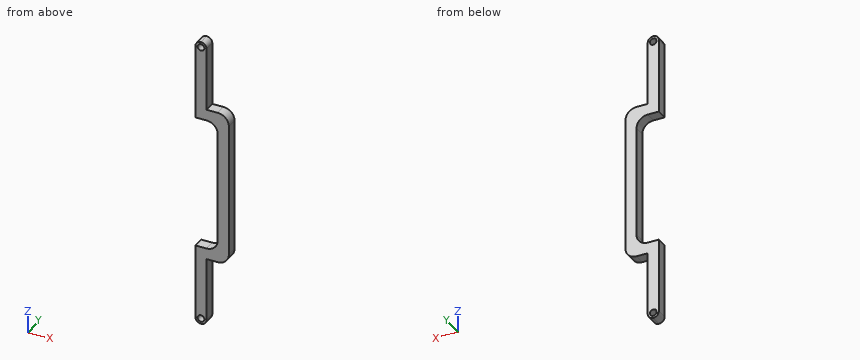
Autodesk Inventor part; units mm, degrees
ref_plane "YZ Plane" through (0, 0, 0) normal (1, 0, 0) x (0, 1, 0)
ref_plane "XZ Plane" through (0, 0, 0) normal (0, 1, 0) x (-1, 0, 0)
ref_plane "XY Plane" through (0, 0, 0) normal (0, 0, 1) x (1, 0, 0)
sketch "Эскиз1" plane through (0, 0, 0) normal (0, 1, 0) x (-1, 0, 0)
  line L0 (0, 0) -> (5, 0)
  line L1 (5, 0) -> (5, -66)
  line L2 (5, -66) -> (0, -66)
  line L3 (0, -66) -> (0, 0)
  line L4 (2.5, 0) -> (2.5, -2.5)
  circle A0 centre (2.5, -2.5) radius 1.5
  line L5 (0, -66) -> (-10, -66)
  line L6 (-10, -66) -> (-10, -31)
  line L7 (-10, -31) -> (0, -31)
  line L8 (0, -31) -> (0, -66)
  line L9 (5, -66) -> (0, -66)
  line L10 (5, -66) -> (-5, -66)
  line L11 (-5, -66) -> (-5, -36)
  line L12 (-5, -36) -> (5, -36)
  line L13 (5, -36) -> (5, -66)
  point P0 (0, -31)
  point P1 (0, -36)
  point P2 (5, -36)
  dimension "d0" = 5
  dimension "d1" = 66
  dimension "d4" = 2.5
  dimension "d5" = 3
  dimension "d7" = 10
  dimension "d8" = 35
  dimension "d11" = 10
  dimension "d12" = 30
extrude "Выдавливание1" add sketch "Эскиз1" along normal blind 5 contours L0 L1 L12 L3 | L3 L12 L11 L5 L6 L7
fillet "Сопряжение1" radius 2.5 2 edges at (0, 2.5, 0) (-5, 2.5, 0)
fillet "Сопряжение2" radius 5 2 edges at (10, 2.5, -31) (5, 2.5, -36)
mirror "Зеркальное отражение2" about plane through (10, 0, -66) normal (0, 0, -1)
equation "\"d11\" = d7"
equation "\"d12\" = d8 - d0"
properties part number "Балка рулевого управления"
Can you work these out from the model? Positions are in its coordinate system, mm. Coordinates: 2 decimals unless noted, no trailing zeros. Write each loop counter-clockwise with the first axis right and the second up, starting at its lowest first coordinate (ties: lowest second). Pieces come first, ordered by that corner, then holes.
Q1. Imagine slicing it at B-B, the plane z = -49. List the corners of the cut face in (x, y) for me, plus the area to 3 significant figures.
Results found:
outline: (5, 0) - (10, 0) - (10, 5) - (5, 5) - close
area: 25.0 mm2
Q2. For P1, Ø1.5, axis at y = 3, z = -112, coming from the +X side; P2, Ø1, axis at x = 4, y = 3, coming from the +Z side; P3, Ø2.5, axis at x = -2.5, z = -2.5, coming from the -Y side; P4, Ø2.5, axis at y = 1.5, z = -59, coming from the -X side, each with a flat end and sliding along its axis, tell me the tip position at first contact or that it passes through.
Results found:
P1: stops at x = 0
P2: stops at z = -31
P3: passes through
P4: stops at x = 5
Q3. Please list where these lines run through material, in increasing order: L1, parallel to Z at x = -2.5, y = 1; L2, parallel to Z at x = 0.5, y = 4; L3, parallel to X at y = 3.9, z = -129.5.
Results found:
L1: z = -132 to -131, -128 to -96, -36 to -4, -1 to 0
L2: z = -101 to -95.97, -36.03 to -31
L3: x = -5 to -4, -1 to 0
Q4. Imagine slicing it at A-A, the plane y = 2. Count the separate pieces of the cut face and the enclosed holes in it, plus the area to 4 significant figures.
Results found:
separate pieces: 1
enclosed holes: 2
area: 740.5 mm2
Q5. Imagine slicing it at C-C, the plane z = -34. List the corners of the cut face in (x, y) for me, plus the area to 3 significant figures.
Results found:
outline: (-5, 0) - (9.58, 0) - (9.58, 5) - (-5, 5) - close
area: 72.9 mm2
